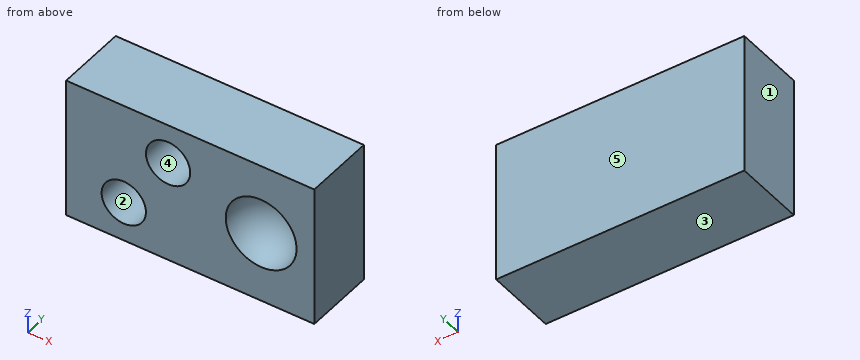
```python
from build123d import *

# Parameters (mm, degrees)
F0_W     = 355.6
F0_H     = 203.2
F0_R     = 31.75
F1_DEPTH = 101.6
F3_DEPTH = 76.2


with BuildPart() as f1:
    # F0 (on Front) → F1 (new body)
    with BuildSketch(Plane.XZ):
        Rectangle(F0_W, F0_H)
        with Locations((-95.25, -44.45)):
            Circle(F0_R, mode=Mode.SUBTRACT)
        with BuildLine():
            ThreePointArc((101.6, 50.8), (152.4, 0), (101.6, -50.8))
            Line((101.6, -50.8), (101.6, 0))
            Line((101.6, 0), (101.6, 50.8))
        make_face(mode=Mode.SUBTRACT)
        with Locations((-31.75, 44.45)):
            Circle(F0_R, mode=Mode.SUBTRACT)
        with BuildLine():
            Line((101.6, 0), (101.6, -50.8))
            ThreePointArc((101.6, -50.8), (152.4, 0), (101.6, 50.8))
            Line((101.6, 50.8), (101.6, 0))
        make_face()
        with Locations((-31.75, 44.45)):
            Circle(F0_R)
        with Locations((-95.25, -44.45)):
            Circle(F0_R)
    extrude(amount=-F1_DEPTH)

    # F0 (on Front) → F2 (revolve, cut)
    with BuildSketch(Plane.XZ):
        with BuildLine():
            Line((101.6, 0), (101.6, -50.8))
            ThreePointArc((101.6, -50.8), (152.4, 0), (101.6, 50.8))
            Line((101.6, 50.8), (101.6, 0))
        make_face()
    revolve(axis=Axis((101.6, 0, 0), (0, 0, 1)), mode=Mode.SUBTRACT)

    # F0 (on Front) → F3 (cut)
    with BuildSketch(Plane.XZ):
        with Locations((-31.75, 44.45)):
            Circle(F0_R)
        with Locations((-95.25, -44.45)):
            Circle(F0_R)
    extrude(amount=-F3_DEPTH, mode=Mode.SUBTRACT)


solid = f1.part
```
The listing builds one solid part. Answer for the finished solid, in the listing's coordinates (mm). Face numbers are marked on the shaded views. A direction names the side the tool comes from. Round coordinates to 2 decimals unless told otherwise and drop trailing zeros. Loops run counter-clockwise (first coordinate to the right, second up) from the corner with the lowest first, then second, coordinate; pieces in that order, holes last. Notation, with made-up numbers: (3, 37.5) - (56, 37.5) arc R32 cw to (56, 76.5) - close; hole circle Ø9 at (41.25, 10.25). An arc over 180 degrees is marked (long way). Use one line per item in the form item = value. Start each with the question number.
1. Consider line 1 (X direction, y = 30, z = -44); line 2 (Z direction, x = -95, y = 16); line 3 (Z direction, x = -31, y = 39). Determine where each line is inside the solid, lowest interval first. Write a range as [from, to].
2. The part is cut by section B-B on x = -31.75. Determine the outline of the cut face in (y, z), then the cut area to 3 significant figures.
3. Given pin 1 Ø19 at (x, z) = (-101.5, -39) entering from -Y, flat-ended and moving along its own axis, determine where the tip first touches the part or whether it passes through.
4. The part is cut by section D-D on y = 7. Determine the outline of the cut face in (x, z), then the cut area to 3 significant figures.
5. The part is cut by section C-C on z = 44.45. Determine the outline of the cut face in (x, y), then the cut area to 3 significant figures.
6. A tool of negligible diameter and unlimited length cuts with its end or side. For the marked faces 4 and 5, from which of +Z, -Z, +X, -X, +Y, -Y can it reach the whole face along a straight path? Write none if from no direction.
7. The part is cut by section A-A on y = 42. Determine the outline of the cut face in (x, z), then the cut area to 3 significant figures.
8. For a pull along X with two mould halves and no side action, classify the marked faces 1, 2 and 3 as pulls with the +X half, pulls with the -X half, needs draft (parallel to the pull), parting line crosses it, or undercut.
Geometry check:
q1.line_1 = [-177.8, -127], [-63.5, 177.8]
q1.line_2 = [-101.6, -76.2], [-12.7, 101.6]
q1.line_3 = [-101.6, 12.71], [76.19, 101.6]
q2.outline = (0, -101.6) - (101.6, -101.6) - (101.6, 101.6) - (0, 101.6) - (0, 76.2) - (76.2, 76.2) - (76.2, 12.7) - (0, 12.7) - close
q2.area = 15,800 mm^2
q3.pin_1 = 76.2
q4.outline = (-177.8, -101.6) - (177.8, -101.6) - (177.8, 101.6) - (-177.8, 101.6) - close; hole circle Ø63.5 at (-95.25, -44.45); hole circle Ø63.5 at (-31.75, 44.45); hole circle Ø100.63 at (101.6, 0)
q4.area = 58,000 mm^2
q5.outline = (-177.8, 0) - (-63.5, 0) - (-63.5, 76.2) - (0, 76.2) - (0, 0) - (77.01, 0) arc R24.59 cw to (126.19, 0) - (177.8, 0) - (177.8, 101.6) - (-177.8, 101.6) - close
q5.area = 30,300 mm^2
q6.face_4 = -Y
q6.face_5 = +Z, -Z, +X, -X, +Y
q7.outline = (-177.8, -101.6) - (177.8, -101.6) - (177.8, 101.6) - (-177.8, 101.6) - close; hole circle Ø63.5 at (-95.25, -44.45); hole circle Ø63.5 at (-31.75, 44.45); hole circle Ø57.15 at (101.6, 0)
q7.area = 63,400 mm^2
q8.face_1 = pulls with the -X half
q8.face_2 = undercut
q8.face_3 = needs draft
